Build history of the part. All positions in model axes, mm. A direction names the side the tool comes from. Give positions to 0.01 mm unless a question says otherwise; leave off trailing zeros. Order: outer loops, then holes, each group sorted by start corner. A loop starts at its lowest first (then second) coordinate and runs counter-clockwise, first axis right, second up. Notation, with made-up numbers: (60.5, -21.5) - (80.5, -21.5) arc R6 cw to (80.5, -11.5) - close; hole circle Ø4 at (-30, 75.5). An arc over 180 degrees is marked (long way). Write each question's results on one line, items separated by ' | '. Start each with the question number.
1) Drop flat-ended pins along their axis: pin 1 Ø4.5 at (x, y) = (1, 1) entering from -Z; pin 2 Ø4 at (x, z) = (5.5, 9) entering from -Y. Give the stop position or say it passes through.
2) Drill centre lines: line 1 along X through (y, z) = (0, 14.5); line 2 along Y through (x, z) = (0, 4.75). Where is each one in solid material? Low to high. Write a range as from..to.
3) Tool access for faces 1 (the face through (1.2, 0, 19.5)), 2 (the face through (-2.814, 0.124, 17.979)), 3 (the face through (-1.735, -1.331, 14.472)): list every direction of +Z, -Z, +X, -X, +Y, -Y with a clear straight run to the whole face (end or side of a thin tool).
4) Cut at C-C on z = 8.75. List the corners of the cut face in (x, y), plus the area to 3 significant figures.
5) Two-plate mould, pull along Y, no slides. Class faces 4 (the face through (-11.99, 0.53, 3.7)), 5 (the face through (-5, 9, 0)), 6 (the face through (-2.17, -9.76, 3.7)): +Y half, -Y half, draft (parallel to the pull), parting line (faces both ways), or undercut.
6) Cut at B-B on z = 17.5. List the corners of the cut face in (x, y).
7) Cut at A-A on x = 0. List the corners of the cut face in (y, z), plus the area to 3 significant figures.
from build123d import *

# Parameters (mm, degrees)
F0_R     = 12
F0_R_2   = 10
F1_DEPTH = 7.5
F2_R     = 12
F3_DEPTH = 5
F3_TAPER = 63
F4_R     = 10
F5_DEPTH = 5
F5_TAPER = 61
F6_R     = 2.1869474725
F6_R_2   = 0.9797612236
F7_DEPTH = 4
F8_R     = 2.8165068541
F8_R_2   = 2.1869474725
F8_R_3   = 0.9797612236
F9_DEPTH = 3


with BuildPart() as f1:
    # F0 (on Top) → F1 (new body)
    with BuildSketch(Plane.XY):
        Circle(F0_R)
        Circle(F0_R_2, mode=Mode.SUBTRACT)
    extrude(amount=F1_DEPTH)

    # F2 (on face) → F3 (join)
    with BuildSketch(Plane.XY.offset(7.5)):
        Circle(F2_R)
    extrude(amount=F3_DEPTH, taper=F3_TAPER)

    # F4 (on face) → F5 (cut)
    with BuildSketch(Plane(origin=(0, 0, 7.5), x_dir=(1, 0, 0), z_dir=(0, 0, -1))):
        Circle(F4_R)
    extrude(amount=-F5_DEPTH, taper=F5_TAPER, mode=Mode.SUBTRACT)

    # F6 (on face) → F7 (join)
    with BuildSketch(Plane.XY.offset(12.5)):
        Circle(F6_R)
        Circle(F6_R_2, mode=Mode.SUBTRACT)
    extrude(amount=F7_DEPTH)

    # F8 (on face) → F9 (join)
    with BuildSketch(Plane.XY.offset(16.5)):
        Circle(F8_R)
        Circle(F8_R_2, mode=Mode.SUBTRACT)
        Circle(F8_R_2)
        Circle(F8_R_3, mode=Mode.SUBTRACT)
    extrude(amount=F9_DEPTH)


solid = f1.part
Results:
1) pin 1: z = 11.01 | pin 2: y = -11.25
2) line 1: -2.19..-0.98, 0.98..2.19 | line 2: -12..-10, 10..12
3) face 1: +Z, +X, -X, +Y, -Y | face 2: +Z | face 3: none
4) outline: circle Ø19.09 at (0, 0); hole circle Ø15.49 at (0, 0) | area: 97.9 mm^2
5) face 4: parting line | face 5: draft | face 6: undercut
6) outline: circle Ø5.63 at (0, 0); hole circle Ø1.96 at (0, 0)
7) outline: (-12, 0) - (-10, 0) - (-10, 7.5) - (-0.98, 12.5) - (-0.98, 19.5) - (-2.82, 19.5) - (-2.82, 16.5) - (-2.19, 16.5) - (-2.19, 12.5) - (-12, 7.5) - close; (0.98, 12.5) - (10, 7.5) - (10, 0) - (12, 0) - (12, 7.5) - (2.19, 12.5) - (2.19, 16.5) - (2.82, 16.5) - (2.82, 19.5) - (0.98, 19.5) - close | area: 66.7 mm^2
